Here's how the part is built. I have some questions about the finished solid (model axes, mm). Round coordinates to 2 decimals unless told otherwise and drop trailing zeros. Loops run counter-clockwise (first coordinate to the right, second up) from the corner with the lowest first, then second, coordinate; pieces in that order, holes last. Notation, with made-up numbers: M 42,89 L 68,89 A11 cw 68,107 Z; hole C 44.5,-29.5 d7. An arc over 180 degrees is marked long. Answer as a JSON object with one key per item and string values.
from build123d import *

# Parameters (mm, degrees)
SKIZZE1_R                       = 2.5
AUFSATZ_LINEAR_AUSTRAGEN1_DEPTH = 1


with BuildPart() as part:
    # Skizze1 → Aufsatz-Linear austragen1 (new body)
    with BuildSketch(Plane(origin=(0, 0, 0), x_dir=(1, 0, 0), z_dir=(0, 1, 0))):
        with BuildLine():
            Line((0, -5.5), (-30, -5.5))
            ThreePointArc((-30, -5.5), (-35.5, 0), (-30, 5.5))
            Line((-30, 5.5), (0, 5.5))
            ThreePointArc((0, 5.5), (5.5, 0), (0, -5.5))
        make_face()
        with Locations(Location((0, 0, 0), (0, 0, 270))):
            Circle(SKIZZE1_R, mode=Mode.SUBTRACT)
        with Locations(Location((-20, 0, 0), (0, 0, 270))):
            Circle(SKIZZE1_R, mode=Mode.SUBTRACT)
        with Locations(Location((-10, 0, 0), (0, 0, 270))):
            Circle(SKIZZE1_R, mode=Mode.SUBTRACT)
        with Locations(Location((-30, 0, 0), (0, 0, 270))):
            Circle(SKIZZE1_R, mode=Mode.SUBTRACT)
    extrude(amount=AUFSATZ_LINEAR_AUSTRAGEN1_DEPTH)


solid = part.part
Item 1: I want a section at A-A, the plane y = 0.3. Please give me the cut outline in (x, z), then the cut area to 3 significant figures.
Resolved:
{"outline": "M -30,-5.5 L 0,-5.5 A5.5 ccw 0,5.5 L -30,5.5 A5.5 ccw Z; hole C -30,0 d5; hole C -20,0 d5; hole C -10,0 d5; hole C 0,0 d5", "area": "346 mm²"}
Item 2: If we mould it in two halves opening along Z, with no side actions, what happens to faces 1 (the face through (-15.2, 0.5, -5.5)), 2 (the face through (-15, 0, 0)), 3 (the face through (5.5, 0.5, -0.1)), 4 (the face through (-2.44, 0.49, -0.54))? For each: pulls with the +Z half, pulls with the -Z half, needs draft (parallel to the pull), parting line crosses it, or undercut.
Resolved:
{"face 1": "pulls with the -Z half", "face 2": "needs draft", "face 3": "parting line crosses it", "face 4": "undercut"}
Item 3: Please list where these lines run through material, in increasing order: probe 1 along X at (y, z) = (0.65, 0); probe 2 along X at (y, z) = (0.6, -0.75); probe 3 along Z at (x, y) = (-11.5, 0.5). Write a range as from..to.
Resolved:
{"probe 1": "-35.5..-32.5, -27.5..-22.5, -17.5..-12.5, -7.5..-2.5, 2.5..5.5", "probe 2": "-35.45..-32.38, -27.62..-22.38, -17.62..-12.38, -7.62..-2.38, 2.38..5.45", "probe 3": "-5.5..-2, 2..5.5"}
Item 4: I want a section at C-C, the plane z = -1.25. Please give me the cut outline in (x, y).
Resolved:
{"outline": "M -35.36,0 L -32.17,0 L -32.17,1 L -35.36,1 Z; M -27.83,0 L -22.17,0 L -22.17,1 L -27.83,1 Z; M -17.83,0 L -12.17,0 L -12.17,1 L -17.83,1 Z; M -7.83,0 L -2.17,0 L -2.17,1 L -7.83,1 Z; M 2.17,0 L 5.36,0 L 5.36,1 L 2.17,1 Z"}
Item 5: I want a section at D-D, the plane x = -20. Please give me the cut outline in (y, z).
Resolved:
{"outline": "M 0,-5.5 L 1,-5.5 L 1,-2.5 L 0,-2.5 Z; M 0,2.5 L 1,2.5 L 1,5.5 L 0,5.5 Z"}
Item 6: I want a section at B-B, the plane x = 1. Please give me the cut outline in (y, z).
Resolved:
{"outline": "M 0,-5.41 L 1,-5.41 L 1,-2.29 L 0,-2.29 Z; M 0,2.29 L 1,2.29 L 1,5.41 L 0,5.41 Z"}
